Answer from the drawing. Dimensions are ordinates in mm from the lowest x, y and z of the part. Coordinates: 2 decimals unless noted, no trailing zeros. Order: outer loops, then holes, each group sorted by start corner. A loop starts at its lowest first (then second) coordinate and runs counter-clockwise, first axis right, second up.
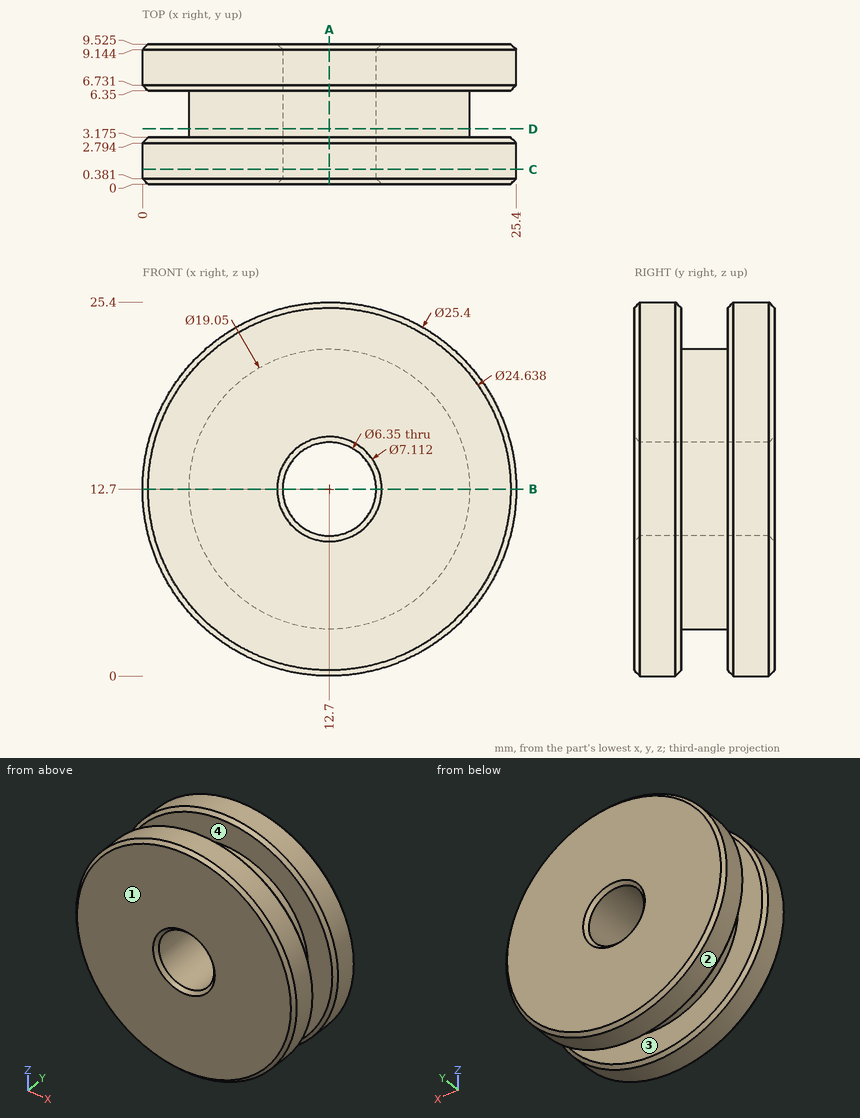
1) Section D-D (y = 3.75) is taken. Give the vertices of the cut face in (x, z) (3 decimals).
2) Consider L1, parallel to Y at x = 7.5, z = 20.75 (3 decimals); L2, parallel to Z at x = 12.7, y = 5 (3 decimals); L3, parallel to Z at x = 12.7, y = 2.75 (3 decimals). Determine where each line is inside the solid, lowest interval first.
3) Section C-C (y = 1) is taken. Give the vertices of the cut face in (x, z) (3 decimals).
4) Section B-B (z = 12.7) is taken. Give the vertices of the cut face in (x, y) (3 decimals), then the cut area to 3 significant figures.
5) Section A-A (x = 12.7) is taken. Give the vertices of the cut face in (y, z) (3 decimals), then the cut area to 3 significant figures.
6) Determine the mould class of the marked faces 1, 2, 3 and 4 for opening direction Y: released by +Y, released by -Y, zero draft, split by the parting line, or undercut.
7) Each of these flat-tipped pins is pushed along its axis until it touches: P1, Ø1, axis at x = 14, y = 8, coming from the -Z side; P2, Ø10, axis at x = 12.7, z = 12.7, coming from the -Y side; P3, Ø2, axis at x = 15, y = 7, coming from the +Z side; P4, Ø3, axis at x = 8.5, y = 5.5, coming from the -Z side. Where does it stop, or does it pass through?
Filled sheet:
1. outline: circle Ø19.05 at (12.7, 12.7); hole circle Ø6.35 at (12.7, 12.7)
2. L1: y = 0 to 3.175, 6.35 to 9.525
2. L2: z = 3.175 to 9.525, 15.875 to 22.225
2. L3: z = 0 to 9.525, 15.875 to 25.4
3. outline: circle Ø25.4 at (12.7, 12.7); hole circle Ø6.35 at (12.7, 12.7)
4. outline: (0, 0.381) - (0.381, 0) - (9.144, 0) - (9.525, 0.381) - (9.525, 9.144) - (9.144, 9.525) - (0.381, 9.525) - (0, 9.144) - (0, 6.731) - (0.381, 6.35) - (3.175, 6.35) - (3.175, 3.175) - (0.381, 3.175) - (0, 2.794) - close; (15.875, 0.381) - (16.256, 0) - (25.019, 0) - (25.4, 0.381) - (25.4, 2.794) - (25.019, 3.175) - (22.225, 3.175) - (22.225, 6.35) - (25.019, 6.35) - (25.4, 6.731) - (25.4, 9.144) - (25.019, 9.525) - (16.256, 9.525) - (15.875, 9.144) - close
4. area: 160 mm2
5. outline: (0, 0.381) - (0.381, 0) - (2.794, 0) - (3.175, 0.381) - (3.175, 3.175) - (6.35, 3.175) - (6.35, 0.381) - (6.731, 0) - (9.144, 0) - (9.525, 0.381) - (9.525, 9.144) - (9.144, 9.525) - (0.381, 9.525) - (0, 9.144) - close; (0, 16.256) - (0.381, 15.875) - (9.144, 15.875) - (9.525, 16.256) - (9.525, 25.019) - (9.144, 25.4) - (6.731, 25.4) - (6.35, 25.019) - (6.35, 22.225) - (3.175, 22.225) - (3.175, 25.019) - (2.794, 25.4) - (0.381, 25.4) - (0, 25.019) - close
5. area: 160 mm2
6. face 1: released by -Y
6. face 2: zero draft
6. face 3: undercut
6. face 4: undercut
7. P1: stops at z = 0.03
7. P2: stops at y = 0
7. P3: stops at z = 25.33
7. P4: stops at z = 0.45
